from build123d import *

# Parameters (mm, degrees)
F1_DEPTH = 2.38125
F2_R     = 2.38125
F3_DEPTH = 25.4
F5_DEPTH = 25.4


with BuildPart() as f1:
    # F0 (on Front) → F1 (new body)
    with BuildSketch(Plane.XZ):
        with BuildLine():
            Line((60.325, 19.05), (7.9375, 19.05))
            ThreePointArc((7.9375, 19.05), (2.32484, 16.72516), (0, 11.1125))
            Line((0, 11.1125), (0, 0))
            Line((0, 0), (9.525, 0))
            Line((9.525, 0), (12.117365, 7.627166))
            ThreePointArc((12.117365, 7.627166), (13.478615, 9.513592), (15.663196, 10.313094))
            Line((15.663196, 10.313094), (60.325, 12.7))
            Line((60.325, 12.7), (60.325, 19.05))
        make_face()
    extrude(amount=F1_DEPTH)

    # F2 (on face) → F3 (cut)
    with BuildSketch(Plane.XZ.offset(2.38125)):
        with Locations((7.9375, 11.1125)):
            Circle(F2_R)
    extrude(amount=-F3_DEPTH, mode=Mode.SUBTRACT)

    # F4 (on face) → F5 (cut)
    with BuildSketch(Plane.XY.offset(19.05)):
        Polygon((60.325, -2.38125), (60.325, -1.190625), (45.24375, -2.38125), align=None)
        Polygon((60.325, 0), (45.24375, 0), (60.325, -1.190625), align=None)
    extrude(amount=-F5_DEPTH, mode=Mode.SUBTRACT)


solid = f1.part
Geometry: final body of the model. Coordinates: model frame, mm. Give positions to 0.01 mm unless a question says otherwise; leave off trailing zeros. Write each loop counter-clockwise with the first axis right and the second up, starting at its lowest first coordinate (ties: lowest second). Pieces come first, ordered by that corner, then holes. Notation, with made-up numbers: M -32.75,23 L 11.25,23 A32 cw 11.25,52 Z; hole C -18,84 d2. An arc over 180 degrees is marked long. Answer in a Markdown table with one row per item. Add a question column.
(1) Section D-D on x = 35.5. Return loops of the section in (y, z).
(2) Mould query, pull axis X, two halves, no side actions, for faces 1 (the flat face through (29, -1, 19.05)), 2 (the flat face through (52.679, -0.587, 15.522)), 3 (the cylindrical face through (6.18, -1.21, 12.72)). Classes: +X half, -X half, draft (parallel to the pull), parting line (faces both ways), or undercut.
(3) Section C-C on z = 5. Return loops of the section in (x, y).
(4) First-contact query: pin 1 (8 mm diameter, centred on x = 40, z = 7.5, fed in from +Y); pin 2 (1 mm diameter, centred on y = -0.5, z = 9, fed in from +X). Flat tips, straight axial feed; report the tip coordinate or a pass-through.
(5) Section A-A on x = 6.5. Return loops of the section in (y, z).
(6) Ray query, line 1 (X direction, y = -1.3, z = 9); line 2 (X direction, y = -0.75, z = 9.75); line 3 (Z direction, x = 15.5, y = -0.6). Return the intervals inside material, ascending.
Result set:
| question | item | result |
|---|---|---|
| 1 | outline | M -2.38,11.37 L 0,11.37 L 0,19.05 L -2.38,19.05 Z |
| 2 | face 1 | draft |
| 2 | face 2 | +X half |
| 2 | face 3 | undercut |
| 3 | outline | M 0,-2.38 L 11.22,-2.38 L 11.22,0 L 0,0 Z |
| 4 | pin 1 | passes through |
| 4 | pin 2 | stops at x = 13.46 |
| 5 | outline | M -2.38,0 L 0,0 L 0,9.21 L -2.38,9.21 Z; M -2.38,13.01 L 0,13.01 L 0,18.92 L -2.38,18.92 Z |
| 6 | line 1 | x = 0 to 6.84, 9.04 to 12.92 |
| 6 | line 2 | x = 0 to 5.98, 9.89 to 13.83 |
| 6 | line 3 | z = 10.3 to 19.05 |
